```python
from build123d import *

# Parameters (mm, degrees)
SKETCH3_R           = 1.5
BOSS_EXTRUDE1_DEPTH = 1.75
BOSS_EXTRUDE2_DEPTH = 3
BOSS_EXTRUDE3_DEPTH = 0.5
SKETCH7_R           = 0.25
CUT_EXTRUDE1_DEPTH  = 0.5


with BuildPart() as part:
    # Sketch3 → Boss-Extrude1 (new body)
    with BuildSketch(Plane(origin=(0, 0, 0), x_dir=(1, 0, 0), z_dir=(0, 1, 0))):
        with BuildLine():
            Line((-16, 18), (16, 18))
            ThreePointArc((16, 18), (17.414213562, 17.414213562), (18, 16))
            Line((18, 16), (18, -16))
            ThreePointArc((18, -16), (17.414213562, -17.414213562), (16, -18))
            Line((16, -18), (-16, -18))
            ThreePointArc((-16, -18), (-17.414213562, -17.414213562), (-18, -16))
            Line((-18, -16), (-18, 16))
            ThreePointArc((-18, 16), (-17.414213562, 17.414213562), (-16, 18))
        make_face()
        with Locations((-15.25, 15.25)):
            Circle(SKETCH3_R, mode=Mode.SUBTRACT)
        with Locations((15.25, 15.25)):
            Circle(SKETCH3_R, mode=Mode.SUBTRACT)
        with Locations((15.25, -15.25)):
            Circle(SKETCH3_R, mode=Mode.SUBTRACT)
        with Locations((-15.25, -15.25)):
            Circle(SKETCH3_R, mode=Mode.SUBTRACT)
    extrude(amount=BOSS_EXTRUDE1_DEPTH)

    # Sketch5 → Boss-Extrude2 (add)
    with BuildSketch(Plane.XY.offset(18)):
        with BuildLine():
            Line((4.049502187, 1.75), (8.049502187, 1.75))
            Line((8.049502187, 1.75), (8.049502187, 3.006518046))
            ThreePointArc((8.049502187, 3.006518046), (7.990923543, 3.147939402), (7.849502187, 3.206518046))
            Line((7.849502187, 3.206518046), (7.559209809, 3.206518046))
            ThreePointArc((7.559209809, 3.206518046), (7.417788453, 3.26509669), (7.359209809, 3.406518046))
            Line((7.359209809, 3.406518046), (7.359209809, 3.55))
            ThreePointArc((7.359209809, 3.55), (7.300631165, 3.691421356), (7.159209809, 3.75))
            Line((7.159209809, 3.75), (4.896173717, 3.75))
            ThreePointArc((4.896173717, 3.75), (4.754752361, 3.691421356), (4.696173717, 3.55))
            Line((4.696173717, 3.55), (4.696173717, 3.406518046))
            ThreePointArc((4.696173717, 3.406518046), (4.637595073, 3.26509669), (4.496173717, 3.206518046))
            Line((4.496173717, 3.206518046), (4.249502187, 3.206518046))
            ThreePointArc((4.249502187, 3.206518046), (4.10808083, 3.147939402), (4.049502187, 3.006518046))
            Line((4.049502187, 3.006518046), (4.049502187, 1.75))
        make_face()
        with BuildLine():
            Line((4.896173717, 3.65), (7.159209809, 3.65))
            ThreePointArc((7.159209809, 3.65), (7.229920487, 3.620710678), (7.259209809, 3.55))
            Line((7.259209809, 3.55), (7.259209809, 3.406518046))
            ThreePointArc((7.259209809, 3.406518046), (7.347077775, 3.194386012), (7.559209809, 3.106518046))
            Line((7.559209809, 3.106518046), (7.849502187, 3.106518046))
            ThreePointArc((7.849502187, 3.106518046), (7.920212865, 3.077228724), (7.949502187, 3.006518046))
            Line((7.949502187, 3.006518046), (7.949502187, 1.85))
            Line((7.949502187, 1.85), (4.149502187, 1.85))
            Line((4.149502187, 1.85), (4.149502187, 3.006518046))
            ThreePointArc((4.149502187, 3.006518046), (4.178791509, 3.077228724), (4.249502187, 3.106518046))
            Line((4.249502187, 3.106518046), (4.496173717, 3.106518046))
            ThreePointArc((4.496173717, 3.106518046), (4.708305751, 3.194386012), (4.796173717, 3.406518046))
            Line((4.796173717, 3.406518046), (4.796173717, 3.55))
            ThreePointArc((4.796173717, 3.55), (4.825463039, 3.620710678), (4.896173717, 3.65))
        make_face(mode=Mode.SUBTRACT)
    extrude(amount=-BOSS_EXTRUDE2_DEPTH)

    # Sketch6 → Boss-Extrude3 (add)
    with BuildSketch(Plane(origin=(0, 0, 15), x_dir=(-1, 0, 0), z_dir=(0, 0, -1))):
        with BuildLine():
            Line((-4.049502187, 1.75), (-4.049502187, 3.006518046))
            ThreePointArc((-4.049502187, 3.006518046), (-4.10808083, 3.147939402), (-4.249502187, 3.206518046))
            Line((-4.249502187, 3.206518046), (-4.496173717, 3.206518046))
            ThreePointArc((-4.496173717, 3.206518046), (-4.637595073, 3.26509669), (-4.696173717, 3.406518046))
            Line((-4.696173717, 3.406518046), (-4.696173717, 3.55))
            ThreePointArc((-4.696173717, 3.55), (-4.754752361, 3.691421356), (-4.896173717, 3.75))
            Line((-4.896173717, 3.75), (-7.159209809, 3.75))
            ThreePointArc((-7.159209809, 3.75), (-7.300631165, 3.691421356), (-7.359209809, 3.55))
            Line((-7.359209809, 3.55), (-7.359209809, 3.406518046))
            ThreePointArc((-7.359209809, 3.406518046), (-7.417788453, 3.26509669), (-7.559209809, 3.206518046))
            Line((-7.559209809, 3.206518046), (-7.849502187, 3.206518046))
            ThreePointArc((-7.849502187, 3.206518046), (-7.990923543, 3.147939402), (-8.049502187, 3.006518046))
            Line((-8.049502187, 3.006518046), (-8.049502187, 1.75))
            Line((-8.049502187, 1.75), (-4.049502187, 1.75))
        make_face()
    extrude(amount=BOSS_EXTRUDE3_DEPTH)

    # Sketch7 → Cut-Extrude1 (cut)
    with BuildSketch(Plane(origin=(0, 0, 14.5), x_dir=(-1, 0, 0), z_dir=(0, 0, -1))):
        with Locations((-6.97797188, 2.378259023)):
            Circle(SKETCH7_R)
        with Locations((-6.17797188, 2.378259023)):
            Circle(SKETCH7_R)
        with Locations((-5.37797188, 2.378259023)):
            Circle(SKETCH7_R)
    extrude(amount=-CUT_EXTRUDE1_DEPTH, mode=Mode.SUBTRACT)


solid = part.part
```
The model under review builds one solid part; all positions refer to its coordinate system, in mm. A direction names the side the tool comes from. Coordinates: 2 decimals unless noted, no trailing zeros. Loops run counter-clockwise (first coordinate to the right, second up) from the corner with the lowest first, then second, coordinate; pieces in that order, holes last. Notation, with made-up numbers: (54, 64.25) -> (72, 64.25) arc R22 ccw to (72, 101.25) -> close; hole circle Ø8 at (36.25, 42). An arc over 180 degrees is marked (long way). Answer as CSV lines item,"result".
Item 1: Take a section at D-D, the plane z = -6.5. State the section outline as (x, y) points, and give its area (3 significant figures).
Results below:
outline,"(-18, 0) -> (18, 0) -> (18, 1.75) -> (-18, 1.75) -> close"
area,"63.0 mm2"
Item 2: Insertion check: pin 1 (2 mm diameter, centred on x = -10, y = 3, fed in from +Z); pin 2 (6 mm diameter, centred on x = -12.5, z = 9.5, fed in from +Y); pin 3 (0.5 mm diameter, centred on x = 5.5, y = 2.5, fed in from +Z); pin 4 (1.3 mm diameter, centred on y = 2.5, z = 17, fed in from +X). Each pin has a flat end and moves straight along its axis. Give the tip position at first contact, or say it passes through.
Results below:
pin 1,"passes through"
pin 2,"stops at y = 1.75"
pin 3,"stops at z = 15"
pin 4,"stops at x = 8.05"
Item 3: For L1, parallel to Z at x = 15.25, y = 0.9; L2, parallel to Z at x = 14, y = 1.4; L3, parallel to X at y = 0.9, z = -15.5, list the stretches that pass through material, from the lowest coordinate up.
Results below:
L1,"z = -18 to -16.75, -13.75 to 13.75, 16.75 to 18"
L2,"z = -18 to -16.08, -14.42 to 14.42, 16.08 to 18"
L3,"x = -18 to -16.73, -13.77 to 13.77, 16.73 to 18"
Item 4: Take a section at C-C, the plane y = 0.95. State the section outline as (x, z) points, and give its area (3 significant figures).
Results below:
outline,"(-18, -16) arc R2 ccw to (-16, -18) -> (16, -18) arc R2 ccw to (18, -16) -> (18, 16) arc R2 ccw to (16, 18) -> (-16, 18) arc R2 ccw to (-18, 16) -> close; hole circle Ø3 at (-15.25, -15.25); hole circle Ø3 at (-15.25, 15.25); hole circle Ø3 at (15.25, -15.25); hole circle Ø3 at (15.25, 15.25)"
area,"1,260 mm2"
Item 5: Draft analysis for pull direction Y (two halves, no side actions). For faces 1 (the flat face through (0, 0, 0)), 2 (the cylindrical face through (-17.43, 0.86, -17.4)), 3 (the flat face through (6, 1.85, 17)), 4 (the flat face through (6, 3, 15)), state which applies: +Y half, -Y half, draft (parallel to the pull), parting line (faces both ways), or undercut.
Results below:
face 1,"-Y half"
face 2,"draft"
face 3,"undercut"
face 4,"undercut"
Item 6: Machinability: for faces 5 (the flat face through (6, 3, 14.5)), 6 (the flat face through (18, 1, 0)), which of the approach directions +Z, -Z, +X, -X, +Y, -Y give a long, thin tool a straight path to every point of the face, cutting with its end or side? Answer none if there is none.
Results below:
face 5,"-Z, +X, -X, +Y"
face 6,"+Z, -Z, +X, +Y, -Y"
Item 7: Take a section at B-B, the plane z = -15.25. State the section outline as (x, y) points.
Results below:
outline,"(-18, 0) -> (-16.75, 0) -> (-16.75, 1.75) -> (-18, 1.75) -> close; (-13.75, 0) -> (13.75, 0) -> (13.75, 1.75) -> (-13.75, 1.75) -> close; (16.75, 0) -> (18, 0) -> (18, 1.75) -> (16.75, 1.75) -> close"
Item 8: Take a section at A-A, the plane x = 15.25. State the section outline as (y, z) points, and give its area (3 significant figures).
Results below:
outline,"(0, -18) -> (1.75, -18) -> (1.75, -16.75) -> (0, -16.75) -> close; (0, -13.75) -> (1.75, -13.75) -> (1.75, 13.75) -> (0, 13.75) -> close; (0, 16.75) -> (1.75, 16.75) -> (1.75, 18) -> (0, 18) -> close"
area,"52.5 mm2"
